The listing builds one solid part. Answer for the finished solid, in the listing's coordinates (mm). Round coordinates to 2 decimals unless told otherwise and drop trailing zeros. Write each loop counter-clockwise with the first axis right and the second up, starting at its lowest first coordinate (ties: lowest second). Pieces come first, ordered by that corner, then holes. Notation, with made-up numbers: (85.5, 9.5) - (117.5, 9.5) arc R10 cw to (117.5, 18.5) - close; hole circle Ø6 at (62.25, 5.5). An arc over 180 degrees is marked (long way). Return JSON: item names as keys, results as strings. Group by question number.
from build123d import *

# Parameters (mm, degrees)
F1_DEPTH = 15
F2_R     = 2.5
F3_DEPTH = 5


with BuildPart() as f1:
    # F0 (on Front) → F1 (new body)
    with BuildSketch(Plane.XZ):
        Polygon((-10, 10), (-100, 10), (-100, -90), (0, -90), (0, -80), (-90, -80), (-90, 0), (0, 0), (0, 100), (-100, 100), (-100, 90), (-10, 90), align=None)
    extrude(amount=F1_DEPTH)

    # F2 (on face) → F3 (join)
    with BuildSketch(Plane.XZ.offset(15)):
        with Locations((-14, -85)):
            Circle(F2_R)
        with Locations((-36, -85)):
            Circle(F2_R)
        with Locations((-56, -85)):
            Circle(F2_R)
        with Locations((-74, -85)):
            Circle(F2_R)
        with Locations((-95, -85)):
            Circle(F2_R)
        with Locations((-95, -64)):
            Circle(F2_R)
        with Locations((-95, -44)):
            Circle(F2_R)
        with Locations((-95, -20)):
            Circle(F2_R)
        with Locations((-95, 5)):
            Circle(F2_R)
        with Locations((-73, 5)):
            Circle(F2_R)
        with Locations((-52, 5)):
            Circle(F2_R)
        with Locations((-28, 5)):
            Circle(F2_R)
        with Locations((-5, 5)):
            Circle(F2_R)
        with Locations((-5, 24)):
            Circle(F2_R)
        with Locations((-5, 41)):
            Circle(F2_R)
        with Locations((-5, 58)):
            Circle(F2_R)
        with Locations((-5, 75)):
            Circle(F2_R)
        with Locations((-5, 95)):
            Circle(F2_R)
        with Locations((-96, 95)):
            Circle(F2_R)
        with Locations((-77, 95)):
            Circle(F2_R)
        with Locations((-54, 95)):
            Circle(F2_R)
        with Locations((-29, 95)):
            Circle(F2_R)
    extrude(amount=F3_DEPTH)


solid = f1.part
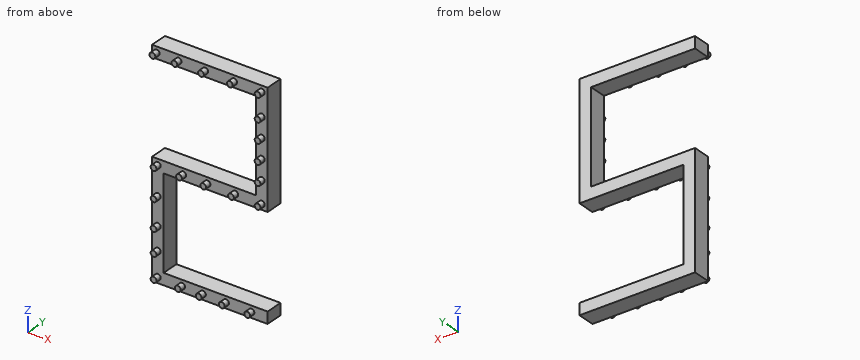
(1) Find section A-A (x = -87). Write down the section's boundary in (y, z).
(2) Find section C-C (y = -11.25). Write down the section's boundary in (x, z), plus the area to 3 significant figures.
(3) Find section B-B (z = -64). Write down the section's boundary in (x, y).
(4) Consider line 1 (Z direction, x = -51, y = -4); line 2 (X direction, y = -11, z = -75); line 3 (Y direction, x = -25, z = 1). Determine where each line is inside the solid, lowest interval first.
(5) A flat-ended cylindrical pin translates along its axis: pin 1 (1 mm diameter, centred on y = -11, z = 14.5, fed in from -X). Find the tip coordinate at first contact, or state that the pin passes through.
Check sheet entries:
{
 "1": {"outline": "(-15, -90) - (0, -90) - (0, -80) - (-15, -80) - close; (-15, 0) - (0, 0) - (0, 10) - (-15, 10) - close; (-15, 90) - (0, 90) - (0, 100) - (-15, 100) - close"},
 "2": {"outline": "(-100, -90) - (0, -90) - (0, -80) - (-90, -80) - (-90, 0) - (0, 0) - (0, 100) - (-100, 100) - (-100, 90) - (-10, 90) - (-10, 10) - (-100, 10) - close", "area": "4,600 mm^2"},
 "3": {"outline": "(-100, -15) - (-97.5, -15) - (-97.5, -20) - (-92.5, -20) - (-92.5, -15) - (-90, -15) - (-90, 0) - (-100, 0) - close"},
 "4": {"line 1": "z = -90 to -80, 0 to 10, 90 to 100", "line 2": "x = -100 to -90", "line 3": "y = -15 to 0"},
 "5": {"pin 1": "stops at x = -10"}
}
